```python
from build123d import *

# Parameters (mm, degrees)
SKETCH2_R           = 20
BOSS_EXTRUDE1_DEPTH = 20
SKETCH3_R           = 30
SKETCH3_R_2         = 20
BOSS_EXTRUDE2_DEPTH = 5


with BuildPart() as part:
    # Sketch2 → Boss-Extrude1 (new body)
    with BuildSketch(Plane(origin=(0, 0, 0), x_dir=(1, 0, 0), z_dir=(0, 1, 0))):
        with BuildLine():
            Line((-14.611492378, -130), (-14.611492378, -103.656657369))
            ThreePointArc((-14.611492378, -103.656657369), (0, -70), (14.611492378, -103.656657369))
            Line((14.611492378, -103.656657369), (14.611492378, -130))
            Line((14.611492378, -130), (54.611492378, -130))
            Line((54.611492378, -130), (54.611492378, -140))
            Line((54.611492378, -140), (100, -140))
            ThreePointArc((100, -140), (128.284271247, -128.284271247), (140, -100))
            Line((140, -100), (140, -54))
            Line((140, -54), (130, -54))
            ThreePointArc((130, -54), (76, 0), (130, 54))
            Line((130, 54), (140, 54))
            Line((140, 54), (140, 100))
            ThreePointArc((140, 100), (128.284271247, 128.284271247), (100, 140))
            Line((100, 140), (54.611492378, 140))
            Line((54.611492378, 140), (54.611492378, 130))
            Line((54.611492378, 130), (14.611492378, 130))
            Line((14.611492378, 130), (14.611492378, 103.656657369))
            ThreePointArc((14.611492378, 103.656657369), (0, 70), (-14.611492378, 103.656657369))
            Line((-14.611492378, 103.656657369), (-14.611492378, 130))
            Line((-14.611492378, 130), (-50, 130))
            Line((-50, 130), (-50, 140))
            Line((-50, 140), (-100, 140))
            ThreePointArc((-100, 140), (-128.284271247, 128.284271247), (-140, 100))
            Line((-140, 100), (-140, 54))
            Line((-140, 54), (-130, 54))
            ThreePointArc((-130, 54), (-76, 0), (-130, -54))
            Line((-130, -54), (-140, -54))
            Line((-140, -54), (-140, -100))
            ThreePointArc((-140, -100), (-128.284271247, -128.284271247), (-100, -140))
            Line((-100, -140), (-50, -140))
            Line((-50, -140), (-50, -130))
            Line((-50, -130), (-14.611492378, -130))
        make_face()
        with Locations(Location((-100, -100, 0), (0, 0, 270))):
            Circle(SKETCH2_R, mode=Mode.SUBTRACT)
        with Locations(Location((-100, 100, 0), (0, 0, 270))):
            Circle(SKETCH2_R, mode=Mode.SUBTRACT)
        with Locations(Location((100, 100, 0), (0, 0, 270))):
            Circle(SKETCH2_R, mode=Mode.SUBTRACT)
        with Locations(Location((100, -100, 0), (0, 0, 270))):
            Circle(SKETCH2_R, mode=Mode.SUBTRACT)
    extrude(amount=BOSS_EXTRUDE1_DEPTH)

    # Sketch3 → Boss-Extrude2 (add)
    # profile 1 of 4: a face of its own
    with BuildSketch(Plane(origin=(0, 20, 0), x_dir=(1, 0, 0), z_dir=(0, 1, 0))):
        with Locations(Location((-100, 100, 0), (0, 0, 270))):
            Circle(SKETCH3_R)
        with Locations(Location((-100, 100, 0), (0, 0, 270))):
            Circle(SKETCH3_R_2, mode=Mode.SUBTRACT)
    # profile 2 of 4: a face of its own
    with BuildSketch(Plane(origin=(0, 20, 0), x_dir=(1, 0, 0), z_dir=(0, 1, 0))):
        with Locations(Location((100, 100, 0), (0, 0, 90))):
            Circle(SKETCH3_R)
        with Locations(Location((100, 100, 0), (0, 0, 90))):
            Circle(SKETCH3_R_2, mode=Mode.SUBTRACT)
    # profile 3 of 4: a face of its own
    with BuildSketch(Plane(origin=(0, 20, 0), x_dir=(1, 0, 0), z_dir=(0, 1, 0))):
        with Locations(Location((100, -100, 0), (0, 0, 270))):
            Circle(SKETCH3_R)
        with Locations(Location((100, -100, 0), (0, 0, 270))):
            Circle(SKETCH3_R_2, mode=Mode.SUBTRACT)
    # profile 4 of 4: a face of its own
    with BuildSketch(Plane(origin=(0, 20, 0), x_dir=(1, 0, 0), z_dir=(0, 1, 0))):
        with Locations(Location((-100, -100, 0), (0, 0, 90))):
            Circle(SKETCH3_R)
        with Locations(Location((-100, -100, 0), (0, 0, 90))):
            Circle(SKETCH3_R_2, mode=Mode.SUBTRACT)
    extrude(amount=BOSS_EXTRUDE2_DEPTH)


solid = part.part
```
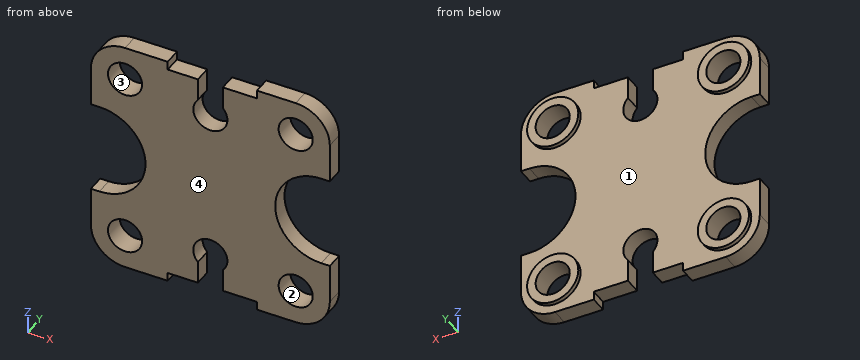
Here's how the part is built. I have some questions about the finished solid (model axes, mm). Face numbers are marked on the shaded views. A direction names the side the tool comes from. Round coordinates to 2 decimals unless told otherwise and drop trailing zeros. Write each loop counter-clockwise with the first axis right and the second up, starting at its lowest first coordinate (ties: lowest second). Pieces come first, ordered by that corner, then holes.
Q1. Will these pins go through, and if not, where does the flat tip stop? P1, Ø5, axis at y = 7.5, z = 21.5, coming from the +X side; P2, Ø4, axis at x = 35.5, y = 12.5, coming from the -Z side; P3, Ø8, axis at y = 13.5, z = -132.5, coming from the -X side; P4, Ø24, axis at x = 0, z = -90, coming from the +Y side.
Q2. If we section it at B-B on x = -96: Write out the boundary of the cut face in (y, z), plus the area to 3 significant figures.
Q3. Which directions (+Z, -Z, +X, -X, +Y, -Y) give clear straight access to the entire face, cutting with the end or side of a thin tool? Please do the marked faces 1 and 2.
Q4. If we section it at C-C on x = 0: Write out the boundary of the cut face in (y, z), plus the area to 3 significant figures.
Q5. Please list where these lines run through material, in increasing order: probe 1 along X at (y, z) = (6.75, 90); probe 2 along X at (y, z) = (19.5, -100); probe 3 along Z at (x, y) = (-97, 9.75).
Q6. If we section it at A-A on z = -86.5: Write out the boundary of the cut face in (x, y), plus the area to 3 significant figures.
Q7. If we mould it in two halves opening along X, with no side actions, what happens to the marked faces 3 and 4? For each: +X half, -X half, draft (parallel to the pull), parting line (faces both ways), or undercut.
Q8. If we section it at D-D on z = 0: Write out the boundary of the cut face in (x, y).
Answer below:
1. P1: stops at x = 81.63
1. P2: stops at z = -130
1. P3: stops at x = -128.07
1. P4: passes through
2. outline: (0, -140) - (20, -140) - (20, -129.73) - (25, -129.73) - (25, -119.6) - (0, -119.6) - close; (0, -80.4) - (25, -80.4) - (25, -70.27) - (20, -70.27) - (20, -41.95) - (0, -41.95) - close; (0, 41.95) - (20, 41.95) - (20, 70.27) - (25, 70.27) - (25, 80.4) - (0, 80.4) - close; (0, 119.6) - (25, 119.6) - (25, 129.73) - (20, 129.73) - (20, 140) - (0, 140) - close
2. area: 2,560 mm2
3. face 1: +Y
3. face 2: +Y, -Y
4. outline: (0, -70) - (20, -70) - (20, 70) - (0, 70) - close
4. area: 2,800 mm2
5. probe 1: x = -140 to -117.32, -82.68 to -20, 20 to 82.68, 117.32 to 140
5. probe 2: x = -140 to -120, -80 to -17.32, 17.32 to 80, 120 to 140
5. probe 3: z = -140 to -119.77, -80.23 to -42.74, 42.74 to 80.23, 119.77 to 140
6. outline: (-140, 0) - (-114.76, 0) - (-114.76, 25) - (-126.79, 25) - (-126.79, 20) - (-140, 20) - close; (-85.24, 0) - (-19.69, 0) - (-19.69, 20) - (-73.21, 20) - (-73.21, 25) - (-85.24, 25) - close; (19.69, 0) - (85.24, 0) - (85.24, 25) - (73.21, 25) - (73.21, 20) - (19.69, 20) - close; (114.76, 0) - (140, 0) - (140, 20) - (126.79, 20) - (126.79, 25) - (114.76, 25) - close
6. area: 3,870 mm2
7. face 3: undercut
7. face 4: draft
8. outline: (-76, 0) - (76, 0) - (76, 20) - (-76, 20) - close
